Geometry check sheet. Reference: the model listing, model coordinates, mm. A direction names the side the tool comes from. Round coordinates to 2 decimals unless told otherwise and drop trailing zeros. Write each loop counter-clockwise with the first axis right and the second up, starting at its lowest first coordinate (ties: lowest second). Pieces come first, ordered by that corner, then holes. Notation, with made-up numbers: M -14.75,64.5 L 34.25,64.5 A24 ccw 34.25,86.5 Z; hole C -14.75,33 d11. An arc over 180 degrees is marked long. Use a Markdown table: item, result.
Autodesk Inventor part; units mm, degrees
ref_plane "YZ Plane" through (0, 0, 0) normal (1, 0, 0) x (0, 1, 0)
ref_plane "XZ Plane" through (0, 0, 0) normal (0, 1, 0) x (-1, 0, 0)
ref_plane "XY Plane" through (0, 0, 0) normal (0, 0, 1) x (1, 0, 0)
sketch "Esquisse1" plane through (0, 0, 0) normal (0, 1, 0) x (-1, 0, 0)
  line L0 (-70.5281, 61.3918) -> (-58.0281, -1.6082)
  line L1 (-58.0281, -1.6082) -> (61.9719, -1.6082)
  line L2 (61.9719, -1.6082) -> (74.4719, 61.3918)
  line L3 (74.4719, 61.3918) -> (-70.5281, 61.3918)
  dimension "d2" = 145
  dimension "d3" = 120
  dimension "d4" = 63
  dimension "d5" = 12.5
extrude "Extrusion1" add sketch "Esquisse1" along normal blind 5
sketch "Esquisse2" plane through (0, 5, 0) normal (0, 1, 0) x (1, 0, 0)
  line L0 (-74.4719, -61.3918) -> (70.5281, -61.3918)
  line L1 (38.0281, -61.3918) -> (28.0281, -1.3918)
  line L2 (28.0281, -1.3918) -> (-31.9719, -1.3918)
  line L3 (-31.9719, -1.3918) -> (-41.9719, -61.3918)
  line L4 (-41.9719, -61.3918) -> (-14.4719, -61.3918)
  line L5 (-14.4719, -61.3918) -> (-14.4719, -53.3918)
  line L6 (-14.4719, -53.3918) -> (10.5281, -53.3918)
  line L7 (10.5281, -53.3918) -> (10.5281, -61.3918)
  line L8 (10.5281, -61.3918) -> (38.0281, -61.3918)
  point P0 (0, 0)
  dimension "d8" = 60
  dimension "d9" = 80
  dimension "d10" = 60
  dimension "d11" = 10
  dimension "d12" = 145
  dimension "d13" = 32.5
  dimension "d14" = 25
  dimension "d15" = 27.5
  dimension "d16" = 8
extrude "Extrusion2" add sketch "Esquisse2" along normal blind 15 contours L3 L2 L1 L0 L7 L6 L5
fillet "Congé1" radius 10 4 edges at (58.0281, 2.5, -1.6082) (-61.9719, 2.5, -1.6082) (-31.9719, 12.5, 1.3918) (28.0281, 12.5, 1.3918)
fillet "Congé2" radius 2 2 edges at (10.5281, 12.5, 53.3918) (-14.4719, 12.5, 53.3918)
sketch "Esquisse3" plane through (0, 20, 0) normal (0, 1, 0) x (1, 0, 0)
  circle A0 centre (-1.9719, -6.3918) radius 1
  line L0 (-14.4719, -61.3918) -> (-14.4719, -55.3918)
  line L1 (10.5281, -55.3918) -> (10.5281, -61.3918)
  line L2 (19.5569, -1.3918) -> (-23.5006, -1.3918)
  point P0 (0, 0)
  dimension "d21" = 2
  dimension "d22" = 25
  dimension "d23" = 12.5
  dimension "d24" = 5
extrude "Extrusion3" cut sketch "Esquisse3" against normal blind 10
sketch "Esquisse4" plane through (19.5569, 5, 1.3918) normal (0, 0, -1) x (-1, 0, 0)
  circle A0 centre (21.5287, 7.5) radius 4
  line L0 (-30.2605, 0) -> (73.3179, 0)
  line L1 (0, 15) -> (43.0575, 15)
  line L2 (61.5287, 0) -> (61.5287, 15)
  line L3 (-18.4713, 0) -> (-18.4713, 15)
  point P0 (19.5569, -5)
  dimension "d27" = 8
  dimension "d28" = 15
  dimension "d29" = 80
  dimension "d30" = 40
  dimension "d31" = 7.5
extrude "Extrusion4" cut sketch "Esquisse4" against normal blind 30
equation "\"d5\" = -0.5 * d3 + 0.5 * d2"
equation "\"d11\" = -0.5 * d10 + 0.5 * d9"
equation "\"d13\" = -0.5 * d9 + 0.5 * d12"
equation "\"d15\" = -0.5 * d14 + 0.5 * d9"
equation "\"d23\" = 0.5 * d22"
equation "\"d30\" = 0.5 * d29"
equation "\"d31\" = 0.5 * d28"
properties part number "Pont arriere" material "Bois (Cerisier)"
Item 1: Material ranges on line 1 along Z through (x, y) = (8.5, 16.5); line 2 along Y through (x, z) = (50.5, 3); line 3 along X through (y, z) = (9.5, 18), recorded low to high. Write a range as from..to.
Outcome:
| item | result |
|---|---|
| line 1 | z = 1.39..53.39 |
| line 2 | y = 0..5 |
| line 3 | x = -34.74..-4.62, 0.67..30.8 |
Item 2: Cross-section at B-B, the plane x = 6. Record the cut outline in (y, z).
Outcome:
| item | result |
|---|---|
| outline | M 0,-1.61 L 5,-1.61 L 5,1.39 L 20,1.39 L 20,53.39 L 5,53.39 L 5,61.39 L 0,61.39 Z |
Item 3: Mould release check, pull along Y, two halves, no side actions. Record for faces 1 (the face through (-68.945, 2.465, 33.534)), 2 (the face through (-1, 0, 30)), 3 (the face through (-2, 13, 31.392)): +Y half, -Y half, draft (parallel to the pull), parting line (faces both ways), or undercut.
Outcome:
| item | result |
|---|---|
| face 1 | draft |
| face 2 | -Y half |
| face 3 | undercut |
Item 4: Cross-section at D-D, the plane z = 39. Record the cut outline in (x, y), and give its area (3 significant figures).
Outcome:
| item | result |
|---|---|
| outline | M -70.03,0 L 66.09,0 L 66.09,5 L 34.3,5 L 34.3,20 L -38.24,20 L -38.24,5 L -70.03,5 Z |
| area | 1,770 mm2 |
Item 5: Cross-section at A-A, the plane y = 12.5. Record the cut outline in (x, z).
Outcome:
| item | result |
|---|---|
| outline | M -41.97,61.39 L -33.36,9.75 A10 ccw -23.5,1.39 L -5.97,1.39 L -5.97,31.39 L 2.03,31.39 L 2.03,1.39 L 19.56,1.39 A10 ccw 29.42,9.75 L 38.03,61.39 L 10.53,61.39 L 10.53,55.39 A2 cw 8.53,53.39 L -12.47,53.39 A2 cw -14.47,55.39 L -14.47,61.39 Z |
Item 6: Access from +Z, -Z, +X, -X, +Y, -Y to the whole of each face (thin tool, end or side, straight path). Record for faces 4 (the face through (-37.61, 12.4, 35.21)), 5 (the face through (26.1, 12.6, 3.83)), 6 (the face through (-14.472, 12, 58)).
Outcome:
| item | result |
|---|---|
| face 4 | -Z, -X, +Y |
| face 5 | -Z, +X, +Y |
| face 6 | +Z, +Y |
Item 7: Cross-section at C-C, the plane z = 19.5. Record the cut outline in (x, y).
Outcome:
| item | result |
|---|---|
| outline | M -66.16,0 L 62.22,0 L 62.22,5 L 31.05,5 L 31.05,20 L -34.99,20 L -34.99,5 L -66.16,5 Z; hole C -1.97,12.5 d8 |
Item 8: Go/stop test with flat-tipped pins: pin 1 (4.5 mm diameter, centred on x = -4.5, y = 15, fed in from +Z); pin 2 (12 mm diameter, centred on y = 3, z = 33.5, fed in from -X); pin 3 (12 mm diameter, centred on y = 15, z = 41, fed in from -X). Record where each tip stops, or that it passes through.
Outcome:
| item | result |
|---|---|
| pin 1 | stops at z = 53.39 |
| pin 2 | stops at x = -70.13 |
| pin 3 | stops at x = -39.57 |
